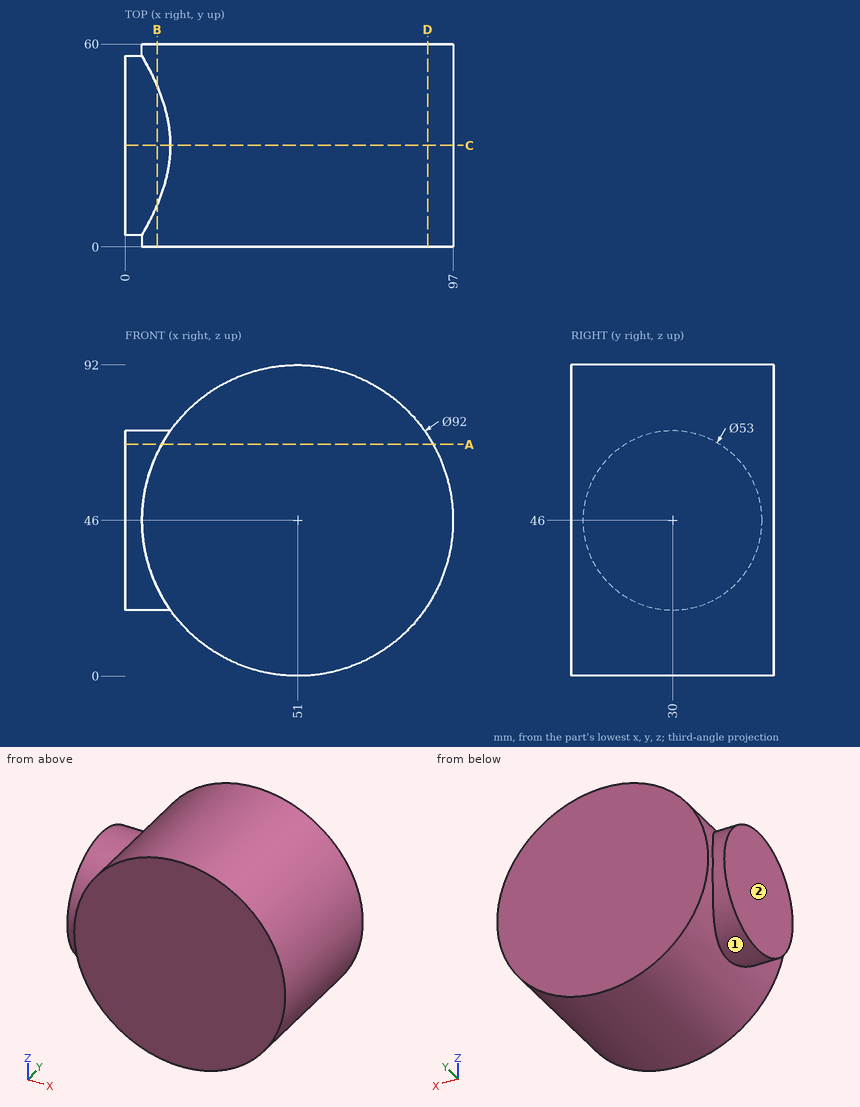
For this review, use the dimensioned drawing (mm, ordinates from the lowest corner) and the shaded views. A direction names the side the tool comes from. Coordinates: 2 decimals unless noted, no trailing zeros. Order: outer loops, then holes, each group sorted by start corner. A loop starts at its lowest first (then second) coordinate and runs counter-clockwise, first axis right, second up. Notation, with made-up numbers: (49, 88.25) - (66, 88.25) arc R6 cw to (66, 99.25) - close; hole circle Ø6 at (42, 84.5). An arc over 180 degrees is marked (long way). Answer as a JSON object with one key per item and string values. Group by question number.
1. We need section C-C on y = 30. State the section outline as (x, z) points, then the cut area to 3 significant figures.
2. For the marked faces 1 and 2, list the 3-axis set-ups (+Z, -Z, +X, -X, +Y, -Y) from which the entire face can be reached by the end or side of a thin tool; tool diameter is ignored.
3. Clearance check with flat-ended pins moving along their axes: P1, Ø5, axis at x = 65, y = 51.5, coming from the -Z side; P2, Ø6, axis at x = 48.5, y = 50, coming from the +Z side; P3, Ø3, axis at x = 56, y = 44.5, coming from the +Z side. State where each tip first meets the part, or that it passes through.
4. We need section D-D on x = 89.5. State the section outline as (y, z) points, then the cut area to 3 significant figures.
5. We need section A-A on z = 68.5. State the section outline as (x, y) points.
6. We need section B-B on x = 9.5. State the section outline as (y, z) points.
7. For probe 1 along X at (y, z) = (32, 26); probe 2 along Z at (x, y) = (60, 10.5); probe 3 along Z at (x, y) = (63.5, 4), list the stretches that pass through material, from the lowest coordinate up.
Final values:
{
 "1": {"outline": "(0, 19.5) - (13.4, 19.5) arc R46 ccw (long way) to (13.4, 72.5) - (0, 72.5) - close", "area": "7,060 mm²"},
 "2": {"face 1": "-X", "face 2": "+Z, -Z, -X, +Y, -Y"},
 "3": {"P1": "z = 1.46", "P2": "z = 92", "P3": "z = 91.87"},
 "4": {"outline": "(0, 20.83) - (60, 20.83) - (60, 71.17) - (0, 71.17) - close", "area": "3,020 mm²"},
 "5": {"outline": "(0, 16) - (10.88, 16) - (10.88, 0) - (91.12, 0) - (91.12, 60) - (10.88, 60) - (10.88, 44) - (0, 44) - close"},
 "6": {"outline": "(0, 26.16) - (12.44, 26.16) arc R26.5 ccw to (47.56, 26.16) - (60, 26.16) - (60, 65.84) - (47.56, 65.84) arc R26.5 ccw to (12.44, 65.84) - (0, 65.84) - close"},
 "7": {"probe 1": "0 to 92.42", "probe 2": "0.89 to 91.11", "probe 3": "1.73 to 90.27"}
}
